Read the model definition and answer for the solid it produces. Units are mm, in the model's axes. Face numbers are marked on the shaded views. Give positions to 0.01 mm unless a question says otherwise; leave off trailing zeros. Loops run counter-clockwise (first coordinate to the right, second up) from the corner with the lowest first, then second, coordinate; pieces in that order, holes last. Notation, with made-up numbers: (81.25, 65) - (121.25, 65) arc R12 ccw to (121.25, 76) - close; hole circle Ø4 at (14.25, 31.5). An arc over 180 degrees is marked (long way). Use a Markdown table: item, result. Add a question column.
Item 1: A cutting plane is placed at A-A (z = 0.85). Determine the outline of the cut face in (x, y).
Item 2: For a pull along X with two mould halves and no side action, classify the marked faces 1, 2 and 3 as +X half, -X half, draft (parallel to the pull), parting line (faces both ways), or undercut.
Item 3: Consider probe 1 along Y at (x, z) = (-0.5, 0.5); probe 2 along Y at (x, z) = (-1.5, 2.65); probe 3 along X at (y, z) = (-0.5, 0.5). Determine where each line is inside the solid, lowest interval first. Write a range as [from, to].
Item 4: A cutting plane is placed at C-C (x = 1.25). Determine the outline of the cut face in (y, z), plus the area to 3 significant figures.
Item 5: A cutting plane is placed at D-D (y = -3). Determine the outline of the cut face in (x, z), plus the area to 3 significant figures.
Item 6: A cutting plane is placed at B-B (y = 0.75). Determine the outline of the cut face in (x, z), plus the area to 3 significant figures.
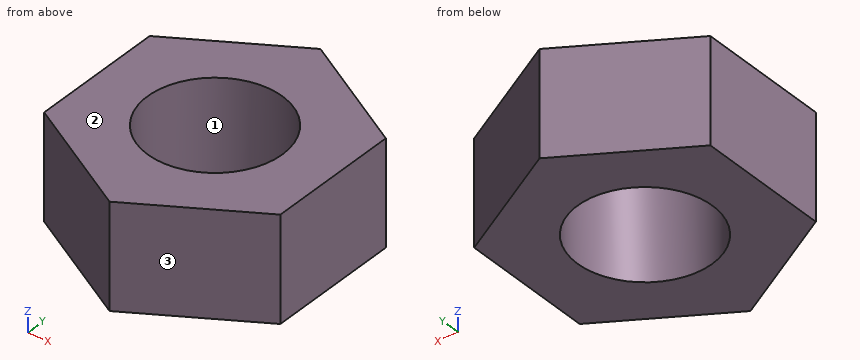
Autodesk Inventor part; units mm, degrees
ref_plane "YZ Plane" through (0, 0, 0) normal (1, 0, 0) x (0, 1, 0)
ref_plane "XZ Plane" through (0, 0, 0) normal (0, 1, 0) x (-1, 0, 0)
ref_plane "XY Plane" through (0, 0, 0) normal (0, 0, 1) x (1, 0, 0)
sketch "Sketch1" plane through (0, 0, 0) normal (0, 0, 1) x (1, 0, 0)
  line L0 (3.5, -2.0347) -> (-0.0121, -4.0484)
  line L1 (-0.0121, -4.0484) -> (-3.5121, -2.0137)
  line L2 (-3.5121, -2.0137) -> (-3.5, 2.0347)
  line L3 (-3.5, 2.0347) -> (0.0121, 4.0484)
  line L4 (0.0121, 4.0484) -> (3.5121, 2.0137)
  line L5 (3.5121, 2.0137) -> (3.5, -2.0347)
  circle A0 centre (0, 0) radius 2
  point P0 (3.5, 0)
  dimension "d0" = 3.5
  dimension "d1" = 4
extrude "Extrusion1" add sketch "Sketch1" along normal blind 3.1
properties part number "m4nut"
Geometry says:
| question | item | result |
|---|---|---|
| 1 | outline | (-3.51, -2.01) - (-0.01, -4.05) - (3.5, -2.03) - (3.51, 2.01) - (0.01, 4.05) - (-3.5, 2.03) - close; hole circle Ø4 at (0, 0) |
| 2 | face 1 | undercut |
| 2 | face 2 | draft |
| 2 | face 3 | +X half |
| 3 | probe 1 | [-3.76, -1.94], [1.94, 3.75] |
| 3 | probe 2 | [-3.18, -1.32], [1.32, 3.18] |
| 3 | probe 3 | [-3.51, -1.94], [1.94, 3.5] |
| 4 | outline | (-3.32, 0) - (-1.56, 0) - (-1.56, 3.1) - (-3.32, 3.1) - close; (1.56, 0) - (3.33, 0) - (3.33, 3.1) - (1.56, 3.1) - close |
| 4 | area | 10.9 mm² |
| 5 | outline | (-1.82, 0) - (1.82, 0) - (1.82, 3.1) - (-1.82, 3.1) - close |
| 5 | area | 11.3 mm² |
| 6 | outline | (-3.5, 0) - (-1.85, 0) - (-1.85, 3.1) - (-3.5, 3.1) - close; (1.85, 0) - (3.51, 0) - (3.51, 3.1) - (1.85, 3.1) - close |
| 6 | area | 10.2 mm² |
